Autodesk Inventor part; units mm, degrees
ref_plane "Work Plane1" through (0, 0, 5) normal (0, 0, 1) x (1, 0, 0)
ref_plane "YZ Plane" through (0, 0, 0) normal (1, 0, 0) x (0, 1, 0)
ref_plane "XZ Plane" through (0, 0, 0) normal (0, 1, 0) x (-1, 0, 0)
sketch "Sketch1" plane through (0, 0, 0) normal (0, 0, 1) x (1, 0, 0)
  circle A0 centre (0, 0) radius 7.5
  circle A1 centre (0, 0) radius 2.5
  dimension "d0" = 15
  dimension "d1" = 5
extrude "Extrusion1" add sketch "Sketch1" along normal blind 10
ref_plane "Work Plane1" through (0, 0, 5) normal (0, 0, 1) x (1, 0, 0)
sketch "Sketch2" plane through (0, 0, 5) normal (0, 0, 1) x (1, 0, 0)
  line L0 (-5.5, -2.6) -> (-3.3, -2.6)
  line L1 (-3.3, -2.6) -> (-3.3, 2.6)
  line L2 (-3.3, 2.6) -> (-5.5, 2.6)
  line L3 (-5.5, 2.6) -> (-5.5, -2.6)
  point P0 (0, 0)
  point P1 (-5.5, 0)
  dimension "d5" = 5.5
  dimension "d6" = 2.2
  dimension "d7" = 5.2
extrude "Extrusion2" cut sketch "Sketch2" along normal blind 5
sketch "Sketch4" plane through (0, 0, 0) normal (1, 0, 0) x (0, 1, 0)
  circle A0 centre (0, 7) radius 1.5
  line L0 (-10.5, 0) -> (10.5, 0)
  point P0 (0, 0)
  dimension "d12" = 3
  dimension "d13" = 7
extrude "Extrusion3" cut sketch "Sketch4" against normal blind 8
sketch "Sketch5" plane through (0, 0, 0) normal (0, 1, 0) x (-1, 0, 0)
  line L0 (7.5, 0) -> (7.5, 10)
  line L1 (7.5, 4) -> (7, 4)
  line L2 (7, 4) -> (7, 10)
  line L3 (7, 10) -> (7.5, 10)
  line L4 (7.5, 10) -> (7.5, 4)
  line L5 (-10.5003, 0) -> (10.5017, 0)
  point P0 (0, 0)
  dimension "d16" = 6
  dimension "d17" = 10
  dimension "d18" = 0.5
extrude "Extrusion4" cut sketch "Sketch5" along normal mid plane 8
properties part number "Acople eje motor"
Could you check a few things on this model? Use its own coordinates, in mm. A direction names the side the tool comes from. Give positions to 0.01 mm unless a question says otherwise; leave off trailing zeros. Order: outer loops, then holes, each group sorted by start corner. A loop starts at its lowest first (then second) coordinate and runs counter-clockwise, first axis right, second up. Notation, with made-up numbers: (8.5, 41.5) - (61.5, 41.5) arc R16 ccw to (61.5, 54.5) - close; hole circle Ø7 at (-3, 33). An arc over 180 degrees is marked (long way). One line per question, with ' | ' between items. Start each with the question number.
Item 1: I need wall thicknesses on probe 1 along X at (y, z) = (0, 4.25); probe 2 along Y at (x, z) = (0, 2.5); probe 3 along X at (y, z) = (-2, 9). Which ranges of each line are inside material? Lowest first, please. Write a range as [from, to].
Item 2: I want a section at D-D on z = 7. Write out the boundary of the cut face in (x, y), then the cut area to 3 significant figures.
Item 3: For faces 1 (the flat face through (-4, -2.6, 7)), 2 (the flat face through (-7, -1.2, 5.6)), 3 (the flat face through (-2, 2, 0)), 4 (the cylindrical face through (2.385, -0.751, 4.93)), 5 (the cylindrical face through (-2.8, -1.2, 6.1)), which set-ups out of +Z, -Z, +X, -X, +Y, -Y let a thin tool reach every point of the face, with its end or its side?
Item 4: I want a section at C-C on z = 3. Write out the boundary of the cut face in (x, y), then the cut area to 3 significant figures.
Item 5: I want a section at A-A on y = 0. Write out the boundary of the cut face in (x, z), then the cut area to 3 significant figures.
Item 6: I'm going to push flat-ended pins straight in: pin 1 Ø2 at (x, z) = (3, 3.5) entering from -Y; pin 2 Ø1.8 at (x, z) = (-4.5, 7.5) entering from +Y; pin 3 Ø2 at (y, z) = (-5, 3) entering from +X. Where does each tip first touch, or does it pass through?
Item 7: I want a section at B-B on x = 0. Write out the boundary of the cut face in (y, z), then the cut area to 3 significant figures.
Item 8: Thinking about a two-plate mould opening in X: for faces 6 (the cylindrical face through (6.93, 2.87, 4.93)), 7 (the flat face through (3, 0, 10)), 8 (the flat face through (-4, 0, 5)), 9 (the flat face through (-4, 2.6, 7)), which applies, pulls with the +X half, pulls with the -X half, needs draft (parallel to the pull), parting line crosses it, or undercut?
Verdict:
1) probe 1: [-7, -2.5], [2.5, 7.5] | probe 2: [-7.5, -2.5], [2.5, 7.5] | probe 3: [-7, -5.5], [-3.3, -1.5], [1.5, 7.23]
2) outline: (-7, -2.69) arc R7.5 ccw (long way) to (-7, 2.69) - (-7, 1.5) - (-5.5, 1.5) - (-5.5, 2.6) - (-3.3, 2.6) - (-3.3, 1.5) - (-2, 1.5) arc R2.5 cw (long way) to (-2, -1.5) - (-3.3, -1.5) - (-3.3, -2.6) - (-5.5, -2.6) - (-5.5, -1.5) - (-7, -1.5) - close | area: 136 mm^2
3) face 1: +Z | face 2: +Z, -X, +Y, -Y | face 3: -Z, +X, -X, +Y, -Y | face 4: +Z, -Z | face 5: -X
4) outline: circle Ø15 at (0, 0); hole circle Ø5 at (0, 0) | area: 157 mm^2
5) outline: (-7.5, 0) - (-2.5, 0) - (-2.5, 5.5) - (-3.3, 5.5) - (-3.3, 5) - (-5.5, 5) - (-5.5, 5.5) - (-7, 5.5) - (-7, 4) - (-7.5, 4) - close; (-7, 8.5) - (-5.5, 8.5) - (-5.5, 10) - (-7, 10) - close; (-3.3, 8.5) - (-2.5, 8.5) - (-2.5, 10) - (-3.3, 10) - close; (2.5, 0) - (7.5, 0) - (7.5, 10) - (2.5, 10) - close | area: 79.1 mm^2
6) pin 1: y = -7.23 | pin 2: y = 6.58 | pin 3: x = 6.34
7) outline: (-7.5, 0) - (-2.5, 0) - (-2.5, 10) - (-7.5, 10) - close; (2.5, 0) - (7.5, 0) - (7.5, 10) - (2.5, 10) - close | area: 100 mm^2
8) face 6: parting line crosses it | face 7: needs draft | face 8: undercut | face 9: undercut
